Study the drawing (mm; zero at the part's minimum x, y, z) and answer. A direction names the side the tool comes from. Coordinates: 2 decimals unless noted, no trailing zeros. Write each loop counter-clockwise with the first axis right and the second up, starting at its lowest first coordinate (ties: lowest second). Pieces come first, ordered by that corner, then holes. Notation, with made-up numbers: (25.5, 16.5) - (69.5, 16.5) arc R26 cw to (69.5, 40.5) - close; hole circle Ø11 at (72.5, 86). An arc over 180 degrees is marked (long way). One line per item, written item: value.
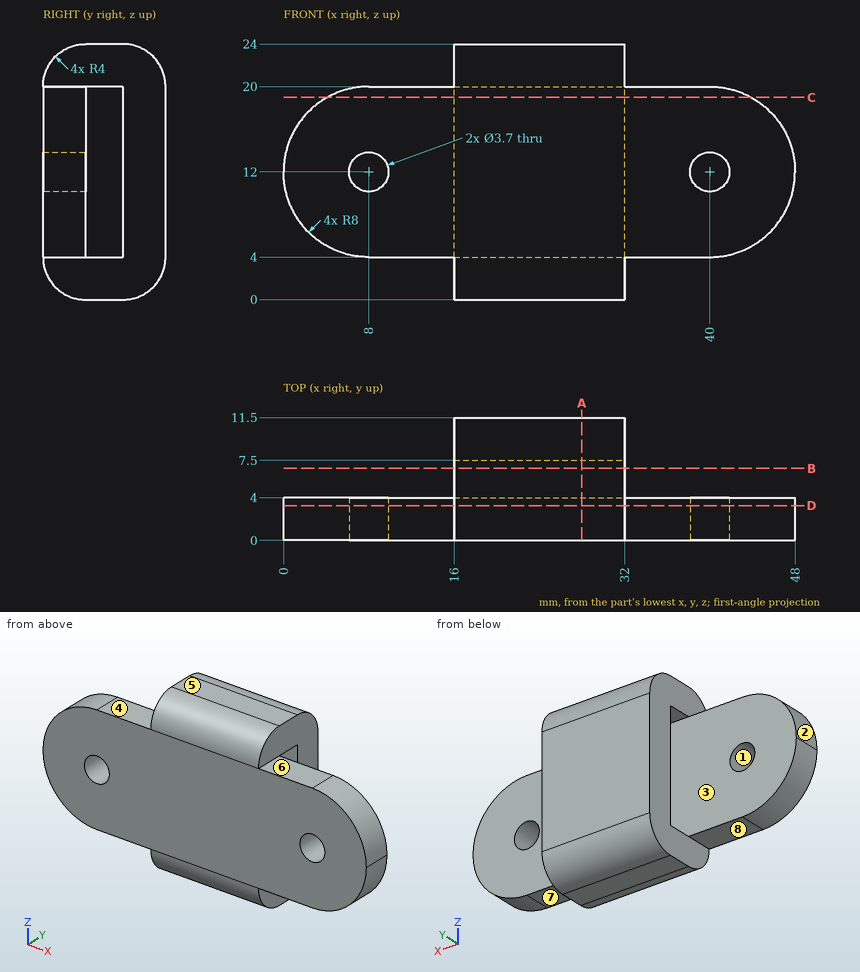
Item 1: Section C-C, the plane z = 19 is taken. Determine the outline of the cut face in (x, y), then the cut area to 3 significant figures.
Evaluation:
outline: (4.13, 0) - (43.87, 0) - (43.87, 4) - (4.13, 4) - close; (16, 7.5) - (32, 7.5) - (32, 11.5) - (16, 11.5) - close
area: 223 mm2
Item 2: Section B-B, the plane y = 6.75 is taken. Determine the outline of the cut face in (x, z), then the cut area to 3 significant figures.
Evaluation:
outline: (16, 0) - (32, 0) - (32, 4) - (16, 4) - close; (16, 20) - (32, 20) - (32, 24) - (16, 24) - close
area: 128 mm2
Item 3: Which of the six approach directions +Z, -Z, +X, -X, +Y, -Y give full straight-line access (tool end or side, diameter ignored) to the marked faces 4, 5, 6, 7 and 8?
Evaluation:
face 4: +Z, -X, +Y, -Y
face 5: +Z, +X, -X, +Y, -Y
face 6: +Z, +X, +Y, -Y
face 7: -Z, +X, +Y, -Y
face 8: -Z, -X, +Y, -Y
Item 4: Section D-D, the plane y = 3.25 is taken. Give the number of separate pieces and of enclosed holes in the cut face, then the cut area to 3 significant figures.
Evaluation:
separate pieces: 1
enclosed holes: 2
area: 817 mm2
Item 5: Section A-A, the plane x = 28 is taken. Determine the outline of the cut face in (y, z).
Evaluation:
outline: (0, 4) arc R4 ccw to (4, 0) - (7.5, 0) arc R4 ccw to (11.5, 4) - (11.5, 20) arc R4 ccw to (7.5, 24) - (4, 24) arc R4 ccw to (0, 20) - close; hole (4, 4) - (7.5, 4) - (7.5, 20) - (4, 20) - close
Item 6: Given pin 1 (1 mm diameter, centred on x = 35, y = 3, fed in from -Z); pin 2 (4 mm diameter, centred on x = 29, y = 1, fed in from -Z); pin 3 (4.5 mm diameter, centred on x = 37.5, y = 2.5, fed in from +Z), each flat-ended and moving along its own axis, determine where each tip first touches the part or whether it passes through.
Evaluation:
pin 1: stops at z = 4
pin 2: stops at z = 0.13
pin 3: stops at z = 20
Item 7: Determine the mould class of the marked faces 1, 2 and 3 for opening direction X: +X half, -X half, draft (parallel to the pull), parting line (faces both ways), or undercut.
Evaluation:
face 1: undercut
face 2: -X half
face 3: draft
Item 8: Consider probe 1 along X at (y, z) = (1.95, 12); probe 2 along Y at (x, z) = (31.5, 17.25); probe 3 along Z at (x, y) = (20, 6). Determine where each line is inside the solid, lowest interval first.
Evaluation:
probe 1: x = 0 to 6.15, 9.85 to 38.15, 41.85 to 48
probe 2: y = 0 to 4, 7.5 to 11.5
probe 3: z = 0 to 4, 20 to 24
